Geometry: final body of the model. Coordinates: model frame, mm. A direction names the side the tool comes from. Coordinates: 2 decimals unless noted, no trailing zeros. Write item = value, one per line.
from build123d import *

# Parameters (mm, degrees)
BOSS_EXTRUDE1_DEPTH             = 40
BOSS_EXTRUDE1_TAPER             = 3
CBORE_FOR_M5_SBHCS1_D           = 5.5
CBORE_FOR_M5_SBHCS1_CBORE_D     = 11
CBORE_FOR_M5_SBHCS1_CBORE_DEPTH = 35


with BuildPart() as part:
    # Sketch1 → Boss-Extrude1 (new body)
    with BuildSketch(Plane(origin=(0, 0, 0), x_dir=(1, 0, 0), z_dir=(0, 1, 0))):
        Polygon((0, 0), (40, 0), (40, 50), (80, 50), (80, 70), (0, 70), align=None)
    extrude(amount=BOSS_EXTRUDE1_DEPTH, taper=BOSS_EXTRUDE1_TAPER)

    # CBORE for M5 SBHCS1 (through all)
    with Locations(Plane(origin=(0, 40, 0), x_dir=(1, 0, 0), z_dir=(0, 1, 0))):
        with Locations((69.508196721, 60), (30, 10), (10, 10), (10, 60), (50.491803279, 60), (30, 60), (10, 30), (30, 30)):
            CounterBoreHole(CBORE_FOR_M5_SBHCS1_D / 2, CBORE_FOR_M5_SBHCS1_CBORE_D / 2, CBORE_FOR_M5_SBHCS1_CBORE_DEPTH)


solid = part.part
1) Pin query (flat end, axial travel): pin 1 (8 mm diameter, centred on x = 37.5, y = 28.5, fed in from +Z); pin 2 (12 mm diameter, centred on x = 52.5, z = -61, fed in from +Y); pin 3 (8 mm diameter, centred on y = 36, z = -46, fed in from -X); pin 4 (5 mm diameter, centred on x = 10, z = -60, fed in from +Y). Return the tip coordinate at first contact, or that it passes through.
Numbers:
pin_1 = -1.28
pin_2 = 40
pin_3 = 1.68
pin_4 = through
2) Set-up query: faces 4 (the face through (50.85, 2.465, -62.727)), 5 (the face through (52, 5, -63)). Return all of +Z, -Z, +X, -X, +Y, -Y with unobstructed straight access to the full face (end or side cutting, diameter ignored); none if empty.
Numbers:
face_4 = +Y, -Y
face_5 = +Y
3) Line query: L1, parallel to X at y = 21, z = -60; L2, parallel to X at y = 27, z = -13; L3, parallel to Z at x = 31.5, y = 13. Output: solid intervals per line, ascending.
Numbers:
L1 = 1.1 to 4.5, 15.5 to 24.5, 35.5 to 44.99, 55.99 to 64.01, 75.01 to 78.9
L2 = 1.42 to 5.39, 14.61 to 25.39, 34.61 to 38.58
L3 = -69.32 to -65.29, -54.71 to -35.29, -24.71 to -15.29, -4.71 to -0.68
4) Mould query, pull axis Z, two halves, no side actions, for faces 1 (the face through (65.454, 22.745, -63.717)), 2 (the face through (30.358, 2.465, -62.727)), 3 (the face through (30, 40, -40)). Classes: pulls with the +Z half, pulls with the -Z half, needs draft (parallel to the pull), parting line crosses it, or undercut.
Numbers:
face_1 = undercut
face_2 = undercut
face_3 = needs draft
5) Section A-A, the plane z = -10. Give the number of separate pieces and of enclosed holes in the cut face, and give its area (3 significant figures).
Numbers:
separate_pieces = 3
enclosed_holes = 0
area = 691 mm²
